CAD build for the part. Positions are in the model's coordinates, mm. A direction names the side the tool comes from. Coordinates: 2 decimals unless noted, no trailing zeros. Order: outer loops, then holes, each group sorted by start corner. A loop starts at its lowest first (then second) coordinate and runs counter-clockwise, first axis right, second up. Notation, with made-up numbers: (19.25, -20.5) - (38.25, -20.5) arc R24 cw to (38.25, 13.5) - close; hole circle Ø5 at (61, 30.5). An arc over 180 degrees is marked (long way). Use one line per item in the form item = value.
```python
from build123d import *

# Parameters (mm, degrees)
SKETCH1_W                                 = 380
SKETCH1_H                                 = 560
BOSS_EXTRUDE1_DEPTH                       = 16
SKETCH2_W                                 = 30
SKETCH2_H                                 = 85
CUT_EXTRUDE1_DEPTH                        = 10
CHAMFER2_SIZE                             = 10
F_8_36_TAPPED_HOLE1_AT_2_COUNT            = 2
F_8_36_TAPPED_HOLE1_AT_2_PITCH            = 31
F_8_36_TAPPED_HOLE1_AT_3_COUNT            = 2
F_8_36_TAPPED_HOLE1_AT_3_PITCH            = 62
LPATTERN1_COUNT                           = 3
LPATTERN1_PITCH                           = 160
CSK_FOR_8_FLAT_HEAD_MACHINE_SCREW_2_COUNT = 2
CSK_FOR_8_FLAT_HEAD_MACHINE_SCREW_2_PITCH = 26


with BuildPart() as part:
    # Sketch1 → Boss-Extrude1 (new body)
    with BuildSketch(Plane(origin=(0, 0, 0), x_dir=(1, 0, 0), z_dir=(0, 1, 0))):
        Rectangle(SKETCH1_W, SKETCH1_H)
    extrude(amount=BOSS_EXTRUDE1_DEPTH)

    # Sketch2 → Cut-Extrude1 (cut)
    with BuildSketch(Plane.XZ):
        with Locations((-175, 160)):
            Rectangle(SKETCH2_W, SKETCH2_H)
        with Locations((-175, 0)):
            Rectangle(SKETCH2_W, SKETCH2_H)
        with Locations((-175, -160)):
            Rectangle(SKETCH2_W, SKETCH2_H)
    extrude(amount=-CUT_EXTRUDE1_DEPTH, mode=Mode.SUBTRACT)

    # Chamfer2
    chamfer2_edges = [part.edges().sort_by_distance(p)[0] for p in [
        (-190, 0, 241.25),
        (-190, 0, 80),
        (-190, 0, -80),
        (-190, 0, -241.25),
    ]]
    chamfer(chamfer2_edges, length=CHAMFER2_SIZE)

    # Sketch5 → #8-36 Tapped Hole1 (revolve, cut)
    with BuildSketch(Plane(origin=(-176, 10, 191), x_dir=(0, 0, -1), z_dir=(1, 0, 0))):
        Polygon((0, 0), (0, 26.037806461), (1.7272, 25), (1.7272, 0), align=None)
    f_8_36_tapped_hole1 = revolve(axis=Axis((-176, 3.65, 191), (0, 1, 0)), mode=Mode.SUBTRACT)

    # #8-36 Tapped Hole1 at 2: #8-36 Tapped Hole1 ×2
    with Locations(*[(0, 0, -i * F_8_36_TAPPED_HOLE1_AT_2_PITCH) for i in range(1, F_8_36_TAPPED_HOLE1_AT_2_COUNT)]):
        add(f_8_36_tapped_hole1, mode=Mode.SUBTRACT)

    # #8-36 Tapped Hole1 at 3: #8-36 Tapped Hole1 ×2
    with Locations(*[(0, 0, -i * F_8_36_TAPPED_HOLE1_AT_3_PITCH) for i in range(1, F_8_36_TAPPED_HOLE1_AT_3_COUNT)]):
        add(f_8_36_tapped_hole1, mode=Mode.SUBTRACT)

    # LPattern1: #8-36 Tapped Hole1 ×3
    with Locations(*[(0, 0, -i * LPATTERN1_PITCH) for i in range(1, LPATTERN1_COUNT)]):
        add(f_8_36_tapped_hole1, mode=Mode.SUBTRACT)

    # LPattern1 copy 1 sketch → LPattern1 copy 1 (revolve, cut)
    with BuildSketch(Plane(origin=(-176, 10, 0), x_dir=(0, 0, -1), z_dir=(1, 0, 0))):
        Polygon((0, 0), (0, 26.037806461), (1.7272, 25), (1.7272, 0), align=None)
    revolve(axis=Axis((-176, 3.65, 0), (0, 1, 0)), mode=Mode.SUBTRACT)

    # LPattern1 copy 2 sketch → LPattern1 copy 2 (revolve, cut)
    with BuildSketch(Plane(origin=(-176, 10, -160), x_dir=(0, 0, -1), z_dir=(1, 0, 0))):
        Polygon((0, 0), (0, 26.037806461), (1.7272, 25), (1.7272, 0), align=None)
    revolve(axis=Axis((-176, 3.65, -160), (0, 1, 0)), mode=Mode.SUBTRACT)

    # LPattern1 copy 3 sketch → LPattern1 copy 3 (revolve, cut)
    with BuildSketch(Plane(origin=(-176, 10, -31), x_dir=(0, 0, -1), z_dir=(1, 0, 0))):
        Polygon((0, 0), (0, 26.037806461), (1.7272, 25), (1.7272, 0), align=None)
    revolve(axis=Axis((-176, 3.65, -31), (0, 1, 0)), mode=Mode.SUBTRACT)

    # LPattern1 copy 4 sketch → LPattern1 copy 4 (revolve, cut)
    with BuildSketch(Plane(origin=(-176, 10, -191), x_dir=(0, 0, -1), z_dir=(1, 0, 0))):
        Polygon((0, 0), (0, 26.037806461), (1.7272, 25), (1.7272, 0), align=None)
    revolve(axis=Axis((-176, 3.65, -191), (0, 1, 0)), mode=Mode.SUBTRACT)

    # Sketch8 → CSK for #8 Flat Head Machine Screw (100)1 (revolve, cut)
    with BuildSketch(Plane(origin=(75, 0, 220), x_dir=(0, 0, -1), z_dir=(1, 0, 0))):
        Polygon((0, 0), (0, 26.350674586), (2.2479, 25), (2.2479, 1.651767624), (4.2164, 0), align=None)
    csk_for_8_flat_head_machine_screw_100 = revolve(axis=Axis((75, -6.35, 220), (0, 1, 0)), mode=Mode.SUBTRACT)

    # CSK for _8 Flat Head Machine Screw _ 2: CSK for #8 Flat Head Machine Screw (100)1 ×2
    with Locations(*[(-i * CSK_FOR_8_FLAT_HEAD_MACHINE_SCREW_2_PITCH, 0, 0) for i in range(1, CSK_FOR_8_FLAT_HEAD_MACHINE_SCREW_2_COUNT)]):
        add(csk_for_8_flat_head_machine_screw_100, mode=Mode.SUBTRACT)

    # Mirror1: CSK for #8 Flat Head Machine Screw (100)1 across plane
    add(csk_for_8_flat_head_machine_screw_100.mirror(Plane.XY), mode=Mode.SUBTRACT)

    # Mirror1 copy 1 sketch → Mirror1 copy 1 (revolve, cut)
    with BuildSketch(Plane(origin=(49, 0, -220), x_dir=(0, 0, 1), z_dir=(1, 0, 0))):
        Polygon((0, 0), (0, -26.350674586), (2.2479, -25), (2.2479, -1.651767624), (4.2164, 0), align=None)
    revolve(axis=Axis((49, -6.35, -220), (0, -1, 0)), mode=Mode.SUBTRACT)


solid = part.part
```
Item 1: Cut at A-A, the plane y = 4.25. Write the cut outline in (x, z).
Derived:
outline = (-184.25, -280) - (190, -280) - (190, 280) - (-184.25, 280) - (-184.25, 202.5) - (-160, 202.5) - (-160, 117.5) - (-184.25, 117.5) - (-184.25, 42.5) - (-160, 42.5) - (-160, -42.5) - (-184.25, -42.5) - (-184.25, -117.5) - (-160, -117.5) - (-160, -202.5) - (-184.25, -202.5) - close; hole circle Ø4.5 at (49, -220); hole circle Ø4.5 at (49, 220); hole circle Ø4.5 at (75, -220); hole circle Ø4.5 at (75, 220)
Item 2: Drop flat-ended pins along their axis: pin 1 (4 mm diameter, centred on x = -176, z = 31, fed in from -Y); pin 2 (5 mm diameter, centred on y = 3, z = -139.5, fed in from -X); pin 3 (2 mm diameter, centred on x = 61, z = 20, fed in from -Y). Give the stop position or say it passes through.
Derived:
pin_1 = 10
pin_2 = -160
pin_3 = 0
Item 3: Drill centre lines: line 1 (X direction, y = 12.45, z = 31); line 2 (X direction, y = 9, z = -161.5); line 3 (X direction, y = 8.5, z = 236). Where is each one in solid material? Low to high. Write a range as [from, to].
Derived:
line_1 = [-190, -177.73], [-174.27, 190]
line_2 = [-160, 190]
line_3 = [-188.5, 190]
Item 4: 3-axis set-ups, long thin cutter, end or side, ignore diameter. For faces 4 (the face through (-172, 10, -159)), 5 (the face through (-3, 16, -4)): which of +Z, -Z, +X, -X, +Y, -Y reach the whole face in a straight line?
Derived:
face_4 = -X, -Y
face_5 = +Z, -Z, +X, -X, +Y
Item 5: Two-plate mould, pull along Z, no slides. Class faces 1 (the face through (-3, 8, 280)), 2 (the face through (-172, 10, 161)), 3 (the face through (2, 0, -4)): +Z half, -Z half, draft (parallel to the pull), parting line (faces both ways), or undercut.
Derived:
face_1 = +Z half
face_2 = undercut
face_3 = draft
